For this review, take the finished solid that the model builds, in its own axes (mm). A direction names the side the tool comes from. Round coordinates to 2 decimals unless told otherwise and drop trailing zeros. Order: outer loops, then holes, each group sorted by start corner. A loop starts at its lowest first (then second) coordinate and runs counter-clockwise, first axis right, second up. Notation, with made-up numbers: M -20.75,78 L 36.25,78 A17 cw 36.25,88 Z; hole C -15,76.5 d1. An arc over 180 degrees is marked long. Put each result on its own line as item: value.
from build123d import *

# Parameters (mm, degrees)
MAIN_POCKETS_DEPTH   = 12
SKETCH2_W            = 34.4
SKETCH2_H            = 54.9
SKETCH2_R            = 1.55
SKETCH2_R_2          = 1.7
SKETCH2_R_3          = 3.125
MOUNTING_HOLES_DEPTH = 3
SKETCH3_R            = 4.6
CUT_EXTRUDE1_DEPTH   = 2
SKETCH4_R            = 1.5
CUT_EXTRUDE2_DEPTH   = 12
SKETCH5_R            = 1.75
CUT_EXTRUDE4_DEPTH   = 3
SKETCH6_W            = 24.4
SKETCH6_H            = 10
CUT_EXTRUDE6_DEPTH   = 3
SKETCH8_R            = 1.7
CUT_EXTRUDE7_DEPTH   = 53.427569083
FILLET1_R            = 1.5
FILLET2_R            = 4.5
FILLET3_R            = 3


with BuildPart() as part:
    # Sketch1 → Main Pockets (new body)
    with BuildSketch(Plane.XY):
        Polygon((17.2, 1.276454737), (17.2, 37.7), (14.2, 37.7), (14.2, 17.7), (4, 17.7), (4, 37.7), (-4, 37.7), (-4, 17.7), (-14.2, 17.7), (-14.2, 37.7), (-17.2, 37.7), (-17.2, 1.276454737), (-17.2, -17.2), (17.2, -17.2), align=None)
        Polygon((-14.2, -14.2), (14.2, -14.2), (14.2, 0), (14.2, 14.7), (4, 14.7), (4, 14.1), (-4, 14.1), (-4, 14.7), (-14.2, 14.7), (-14.2, 0), align=None, mode=Mode.SUBTRACT)
    extrude(amount=-MAIN_POCKETS_DEPTH)

    # Sketch2 → Mounting Holes (add)
    with BuildSketch(Plane.XY):
        with Locations((0, 10.25)):
            Rectangle(SKETCH2_W, SKETCH2_H)
        with Locations((0, -6)):
            Circle(SKETCH2_R, mode=Mode.SUBTRACT)
        with Locations((-5.196152423, 3)):
            Circle(SKETCH2_R, mode=Mode.SUBTRACT)
        with Locations((5.196152423, 3)):
            Circle(SKETCH2_R, mode=Mode.SUBTRACT)
        with Locations((-9.1, 32.7)):
            Circle(SKETCH2_R_2, mode=Mode.SUBTRACT)
        with Locations((9.1, 32.7)):
            Circle(SKETCH2_R_2, mode=Mode.SUBTRACT)
        Circle(SKETCH2_R_3, mode=Mode.SUBTRACT)
    extrude(amount=MOUNTING_HOLES_DEPTH)

    # Sketch3 → Cut-Extrude1 (cut)
    with BuildSketch(Plane.XY):
        Circle(SKETCH3_R)
    extrude(amount=CUT_EXTRUDE1_DEPTH, mode=Mode.SUBTRACT)

    # Sketch4 → Cut-Extrude2 (cut)
    with BuildSketch(Plane(origin=(0, 0, -12), x_dir=(-1, 0, 0), z_dir=(0, 0, -1))):
        with Locations((-14.2, 17.7)):
            Circle(SKETCH4_R)
        with Locations((-4, 17.7)):
            Circle(SKETCH4_R)
        with Locations((4, 17.7)):
            Circle(SKETCH4_R)
        with Locations((14.2, 17.7)):
            Circle(SKETCH4_R)
    extrude(amount=-CUT_EXTRUDE2_DEPTH, mode=Mode.SUBTRACT)

    # Sketch5 → Cut-Extrude4 (cut)
    with BuildSketch(Plane(origin=(0, 17.7, 0), x_dir=(1, 0, 0), z_dir=(0, 1, 0))):
        with Locations(Location((-9.1, 5, 0), (0, 0, 270))):
            Circle(SKETCH5_R)
        with Locations(Location((9.1, 5, 0), (0, 0, 270))):
            Circle(SKETCH5_R)
    extrude(amount=-CUT_EXTRUDE4_DEPTH, mode=Mode.SUBTRACT)

    # Sketch6 → Cut-Extrude6 (cut)
    with BuildSketch(Plane.XZ.offset(17.2)):
        with Locations((0, -7)):
            Rectangle(SKETCH6_W, SKETCH6_H)
    extrude(amount=-CUT_EXTRUDE6_DEPTH, mode=Mode.SUBTRACT)

    # Sketch8 → Cut-Extrude7 (cut, through all)
    with BuildSketch(Plane(origin=(17.2, 0, 0), x_dir=(0, 0, -1), z_dir=(1, 0, 0))):
        with Locations((5, 32.7)):
            Circle(SKETCH8_R)
    extrude(amount=-CUT_EXTRUDE7_DEPTH, mode=Mode.SUBTRACT)

    # Fillet1
    # the kernel refuses this fillet: 1.5 mm, written as the material it adds along each edge
    with BuildSketch(Plane(origin=(-4, 14.7, 3), x_dir=(0, -1, 0), z_dir=(0, 0, -1))) as fillet1_piece_1:
        with BuildLine():
            CenterArc((1.5, 1.2), FILLET1_R, 180, 53.130102354)
            Line((0, 1.2), (0, 0))
            Line((0, 0), (0.6, 0))
        make_face()
    extrude(amount=15)
    with BuildSketch(Plane(origin=(4, 14.7, 3), x_dir=(1, 0, 0), z_dir=(0, 0, -1))) as fillet1_piece_2:
        with BuildLine():
            CenterArc((1.2, 1.5), FILLET1_R, 216.869897646, 53.130102354)
            Line((0, 0.6), (0, 0))
            Line((0, 0), (1.2, 0))
        make_face()
    extrude(amount=15)
    with BuildSketch(Plane(origin=(-14.2, -14.2, 0), x_dir=(1, 0, 0), z_dir=(0, 0, -1))) as fillet1_piece_3:
        with BuildLine():
            CenterArc((FILLET1_R, -FILLET1_R), FILLET1_R, 90, 90)
            Line((0, -FILLET1_R), (0, 0))
            Line((0, 0), (FILLET1_R, 0))
        make_face()
    extrude(amount=12)
    with BuildSketch(Plane(origin=(-14.2, 14.7, 0), x_dir=(1, 0, 0), z_dir=(0, 0, -1)), Plane(origin=(14.2, 14.7, 0), x_dir=(0, -1, 0), z_dir=(0, 0, -1)), Plane(origin=(14.2, -14.2, 0), x_dir=(-1, 0, 0), z_dir=(0, 0, -1))) as fillet1_piece_4:
        with BuildLine():
            CenterArc((FILLET1_R, FILLET1_R), FILLET1_R, 180, 90)
            Line((0, FILLET1_R), (0, 0))
            Line((0, 0), (FILLET1_R, 0))
        make_face()
    extrude(amount=12)

    # Fillet2
    fillet2_edges = [part.edges().sort_by_distance(p)[0] for p in [
        (17.2, -17.2, -4.5),
        (-17.2, -17.2, -4.5),
    ]]
    fillet(fillet2_edges, radius=FILLET2_R)

    # Fillet3
    fillet3_edges = [part.edges().sort_by_distance(p)[0] for p in [
        (-12.2, -15.7, -2),
        (12.2, -15.7, -2),
    ]]
    fillet(fillet3_edges, radius=FILLET3_R)


solid = part.part
(1) To check wall thickness, follow L1, parallel to Y at x = 0, z = 2.3 (3 decimals); L2, parallel to X at y = 23.5, z = -7; L3, parallel to X at y = -8, z = -3.5. State the ranges of each line that lie inside material, in increasing order.
A:
L1: y = -17.2 to -7.55, -4.45 to -3.125, 3.125 to 37.7
L2: x = -17.2 to -14.2, -4 to 4, 14.2 to 17.2
L3: x = -17.2 to -14.2, 14.2 to 17.2
(2) Add section A-A on x = 0. Give the boundary of the cut face in (y, z) (3 decimals), then the cut area to 3 significant figures.
A:
outline: M -17.2,-2 L -14.2,-2 L -14.2,0 L -7.55,0 L -7.55,3 L -17.2,3 Z; M -4.45,2 L -3.125,2 L -3.125,3 L -4.45,3 Z; M 3.125,2 L 4.6,2 L 4.6,0 L 14.1,0 L 14.1,-12 L 37.7,-12 L 37.7,3 L 3.125,3 Z; hole C 32.7,-5 d3.4
area: 411 mm2
(3) Add section C-C on y = 29. Give the boundary of the cut face in (x, z), then the cut area to 3 significant figures.
A:
outline: M -17.2,-12 L -14.2,-12 L -14.2,0 L -4,0 L -4,-12 L 4,-12 L 4,0 L 14.2,0 L 14.2,-12 L 17.2,-12 L 17.2,3 L -17.2,3 Z
area: 271 mm2
(4) Add section D-D on x = 10. Give the boundary of the cut face in (y, z).
A:
outline: M -17.2,-2.11 L -14.2,-2.11 L -14.2,0 L 14.7,0 L 14.7,-3.5 L 17.7,-3.5 L 17.7,0 L 31.26,0 L 31.26,3 L -17.2,3 Z; M 14.7,-12 L 17.7,-12 L 17.7,-6.5 L 14.7,-6.5 Z; M 34.14,0 L 37.7,0 L 37.7,3 L 34.14,3 Z
(5) Draft analysis for pull direction Z (two halves, no side actions). For faces 1 (the face through (3.954, -2.351, 0.986)), 2 (the face through (15.721, 34.386, -4.779)), 3 (the face through (0, -16, -2)), 4 (the face through (7.39, 16.22, -5.38)), state which applies: released by +Z, released by -Z, zero draft, split by the parting line, or undercut.
A:
face 1: zero draft
face 2: undercut
face 3: released by -Z
face 4: undercut
(6) Insertion check: pin 1 Ø4.5 at (x, z) = (9.1, -5) entering from +Y; pin 2 Ø7.5 at (x, y) = (-2.5, -0.5) entering from -Z; pin 3 Ø1.5 at (y, z) = (-15.5, -7) entering from +X. Each pin has a flat end and moves straight along its axis. Give the tip position at first contact, or say it passes through.
A:
pin 1: stops at y = 17.7
pin 2: stops at z = 0
pin 3: stops at x = 16.71
(7) For faces 5 (the face through (11.34, -15.68, -2.9)), 6 (the face through (-9, 17.7, -7)), 7 (the face through (0, 16, -12)), 8 (the face through (2.975, 16.605, -6.084)), list the 3-axis set-ups (+Z, -Z, +X, -X, +Y, -Y) from which the entire face can be reached by the end or side of a thin tool; tool diameter is ignored.
A:
face 5: -Z, -Y
face 6: -Z, +Y
face 7: -Z, +X, -X, +Y, -Y
face 8: -Z
